Source: CAD feature listing. Evaluate the final solid. Frame: model axes, mm. Face numbers are marked on the shaded views. A direction names the side the tool comes from. Round coordinates to 2 decimals unless told otherwise and drop trailing zeros. Order: outer loops, then holes, each group sorted by start corner. A loop starts at its lowest first (then second) coordinate and runs counter-clockwise, first axis right, second up. Notation, with made-up numbers: (13, -7.5) - (43, -7.5) arc R22 ccw to (43, 7.5) - close; hole circle Ø10 at (20.25, -19). An arc over 180 degrees is marked (long way). Put each result on its own line as item: value. Start each with the question number.
1) Contact query for flat-ended pins moving along their axis: P1, Ø4, axis at x = 32.01, z = 2.25, coming from the +Y side; P2, Ø1.5, axis at x = 24, y = 5, coming from the +Z side; P3, Ø1.2, axis at x = 7, y = 2.5, coming from the +Z side; P4, Ø3, axis at x = 32.01, z = 21.45, coming from the -Y side. Output: stop coordinate, or through.
2) Section D-D on z = 16.25. Output: boundary loops of the cut face in (x, y), then the cut area to 3 significant figures.
3) Line query: probe 1 along Z at (x, y) = (32.01, 0.85); probe 2 along X at (y, z) = (0.85, 2.25); probe 3 along Y at (x, z) = (17.5, 2). Output: solid intervals per line, ascending. Write a range as [from, to].
4) Section B-B on x = 32.5. Output: boundary loops of the cut face in (y, z).
5) Section A-A on z = 21.45. Output: boundary loops of the cut face in (x, y), then the cut area to 3 significant figures.
6) Access query for the marked faces 1, 2 and 3. Directions: +Z, -Z, +X, -X, +Y, -Y. A direction counts if a zero-diameter tool reaches every point of the face in a straight line with its end or side. Return the directions, or none.
7) Section C-C on x = 21.85. Output: boundary loops of the cut face in (y, z).
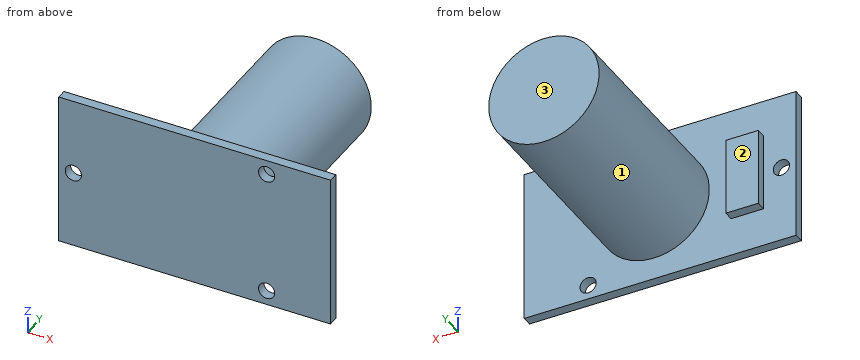
```python
from build123d import *

# Parameters (mm, degrees)
SKETCH2_W           = 41.85
SKETCH2_H           = 23.7
SKETCH2_R           = 1.25
SKETCH2_R_2         = 8.5
BOSS_EXTRUDE1_DEPTH = 1.5
SKETCH2_3_R         = 8.5
BOSS_EXTRUDE2_DEPTH = 33
SKETCH2_6_W         = 5
SKETCH2_6_H         = 12
BOSS_EXTRUDE3_DEPTH = 3


with BuildPart() as part:
    # Sketch2 → Boss-Extrude1 (new body)
    with BuildSketch(Plane(origin=(0, 0, 0), x_dir=(1, 0, 0), z_dir=(0, 1, 0))):
        with Locations((20.925, -11.85)):
            Rectangle(SKETCH2_W, SKETCH2_H)
        with Locations((32.01, -2.25)):
            Circle(SKETCH2_R, mode=Mode.SUBTRACT)
        with Locations((21.85, -11.902335017)):
            Circle(SKETCH2_R_2, mode=Mode.SUBTRACT)
        with Locations((32.01, -21.45)):
            Circle(SKETCH2_R, mode=Mode.SUBTRACT)
        with Locations((2.249488742, -11.897962459)):
            Circle(SKETCH2_R, mode=Mode.SUBTRACT)
    extrude(amount=BOSS_EXTRUDE1_DEPTH)

    # Sketch2<3> → Boss-Extrude2 (add)
    with BuildSketch(Plane(origin=(0, 0, 0), x_dir=(1, 0, 0), z_dir=(0, 1, 0))):
        with Locations((21.85, -11.902335017)):
            Circle(SKETCH2_3_R)
    extrude(amount=BOSS_EXTRUDE2_DEPTH)

    # Sketch2<6> → Boss-Extrude3 (add)
    with BuildSketch(Plane(origin=(0, 0, 0), x_dir=(1, 0, 0), z_dir=(0, 1, 0))):
        with Locations((7.5, -12)):
            Rectangle(SKETCH2_6_W, SKETCH2_6_H)
    extrude(amount=BOSS_EXTRUDE3_DEPTH)


solid = part.part
```
Answer sheet:
1. P1: y = 1.5
1. P2: z = 20.29
1. P3: z = 18
1. P4: y = 0
2. outline: (0, 0) - (41.85, 0) - (41.85, 1.5) - (29.15, 1.5) - (29.15, 33) - (14.55, 33) - (14.55, 1.5) - (10, 1.5) - (10, 3) - (5, 3) - (5, 1.5) - (0, 1.5) - close
2. area: 530 mm^2
3. probe 1: [0, 1], [3.5, 20.2], [22.7, 23.7]
3. probe 2: [0, 30.76], [33.26, 41.85]
3. probe 3: [0, 1.5]
4. outline: (0, 0) - (1.5, 0) - (1.5, 1.1) - (0, 1.1) - close; (0, 3.4) - (1.5, 3.4) - (1.5, 20.3) - (0, 20.3) - close; (0, 22.6) - (1.5, 22.6) - (1.5, 23.7) - (0, 23.7) - close
5. outline: (0, 0) - (30.76, 0) - (30.76, 1.5) - (0, 1.5) - close; (33.26, 0) - (41.85, 0) - (41.85, 1.5) - (33.26, 1.5) - close
5. area: 59.0 mm^2
6. face 1: +Y
6. face 2: +Z, -Z, -X, +Y
6. face 3: +Z, -Z, +X, -X, +Y
7. outline: (0, 0) - (1.5, 0) - (1.5, 3.4) - (33, 3.4) - (33, 20.4) - (1.5, 20.4) - (1.5, 23.7) - (0, 23.7) - close
